Autodesk Fusion 360 part; units mm, degrees
sketch "Sketch1" plane through (0, 0, 0) normal (0, 0, 1) x (1, 0, 0)
  line L0 (-27.5, 0) -> (-12.5, 0)
  line L1 (-12.5, 0) -> (-12.5, 14.8)
  line L2 (-12.5, 14.8) -> (0, 14.8)
  line L3 (0, 31) -> (0, -29)
  line L4 (27.5, 0) -> (12.5, 0)
  line L5 (12.5, 0) -> (12.5, 14.8)
  line L6 (12.5, 14.8) -> (0, 14.8)
  line L7 (-27.5, 4) -> (-16.5, 4)
  line L8 (-16.5, 4) -> (-16.5, 18.8)
  line L9 (-16.5, 18.8) -> (0, 18.8)
  line L10 (16.5, 18.8) -> (0, 18.8)
  line L11 (16.5, 4) -> (16.5, 18.8)
  line L12 (27.5, 4) -> (16.5, 4)
  line L13 (27.5, 4) -> (27.5, 0)
  line L14 (-27.5, 4) -> (-27.5, 0)
  dimension "d2" = 4
  dimension "d3" = 15
  dimension "d4" = 25
  dimension "d5" = 14.8
extrude "Extrude1" add sketch "Sketch1" along normal blind 8
hole "Hole1" at (22.4998, 0, 3.8936) direction (0, 1, 0) diameter 4 depth 5 tip angle 118
hole "Hole2" at (-22.5548, 0, 4.1194) direction (0, 1, 0) diameter 4 depth 5 tip angle 118
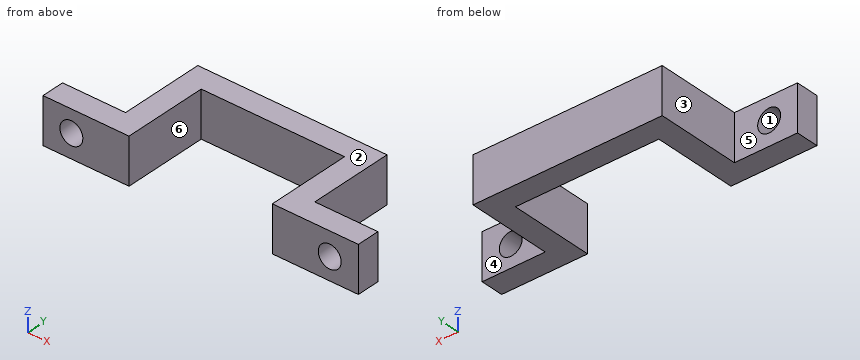
Verification items for the finished model (mm, model axes). Face numbers are marked on the shaded views. A direction names the side the tool comes from. Round coordinates to 2 decimals unless told otherwise and drop trailing zeros. Order: outer loops, then holes, each group sorted by start corner. A loop starts at its lowest first (then second) coordinate and runs counter-clockwise, first axis right, second up. Notation, with made-up numbers: (17.25, 70) - (24.25, 70) arc R8 cw to (24.25, 74) - close; hole circle Ø10 at (21.5, 25.5). An arc over 180 degrees is marked (long way). Use CSV: the item, a comma, the result in double quotes. Start each with the question number.
1) Go/stop test with flat-tipped pins: P1, Ø2.5, axis at x = 1, z = 5.5, coming from the -Y side; P2, Ø1.5, axis at x = 20, z = 6, coming from the +Y side; P3, Ø4, axis at y = 7.5, z = 4.5, coming from the +X side. Record where each tip stops, or that it passes through.
2) Access from +Z, -Z, +X, -X, +Y, -Y to the whole of each face (thin tool, end or side, straight path). Record for the marked faces 4, 5 and 6.
3) Thickness scan on L1, parallel to X at y = 6.5, z = 7.5; L2, parallel to X at y = 2.5, z = 7; L3, parallel to X at y = 1, z = 5.25. Record the ranges inside material, lowest first.
4) Section check A-A, the plane y = 7. Record the cut outline in (x, z), plus the area to 3 significant figures.
5) Section check D-D, the plane z = 3.5. Record the cut outline in (x, y).
6) Section check C-C, the plane x = 23.5. Record the cut outline in (y, z).
7) Section check B-B, the plane y = 1.5. Record the cut outline in (x, z).
8) Mould release check, pull along X, two halves, no side actions. Record for the marked faces 1, 2 and 3: +X half, -X half, draft (parallel to the pull), parting line (faces both ways), or undercut.
Answers:
1,P1,"stops at y = 14.8"
1,P2,"stops at y = 4"
1,P3,"stops at x = 16.5"
2,face 4,"+Z, -Z, +X, +Y"
2,face 5,"+Z, -Z, -X, +Y"
2,face 6,"+Z, -Z, -Y"
3,L1,"x = -16.5 to -12.5, 12.5 to 16.5"
3,L2,"x = -27.5 to -12.5, 12.5 to 27.5"
3,L3,"x = -27.5 to -24.2, -20.91 to -12.5, 12.5 to 21.03, 23.97 to 27.5"
4,outline,"(-16.5, 0) - (-12.5, 0) - (-12.5, 8) - (-16.5, 8) - close; (12.5, 0) - (16.5, 0) - (16.5, 8) - (12.5, 8) - close"
4,area,"64.0 mm²"
5,outline,"(-27.5, 0) - (-24.46, 0) - (-24.46, 4) - (-27.5, 4) - close; (-20.65, 0) - (-12.5, 0) - (-12.5, 14.8) - (12.5, 14.8) - (12.5, 0) - (20.54, 0) - (20.54, 4) - (16.5, 4) - (16.5, 18.8) - (-16.5, 18.8) - (-16.5, 4) - (-20.65, 4) - close; (24.46, 0) - (27.5, 0) - (27.5, 4) - (24.46, 4) - close"
6,outline,"(0, 0) - (4, 0) - (4, 2.16) - (0, 2.16) - close; (0, 5.63) - (4, 5.63) - (4, 8) - (0, 8) - close"
7,outline,"(-27.5, 0) - (-12.5, 0) - (-12.5, 8) - (-27.5, 8) - close; (12.5, 0) - (27.5, 0) - (27.5, 8) - (12.5, 8) - close; hole circle Ø4 at (-22.55, 4.12); hole circle Ø4 at (22.5, 3.89)"
8,face 1,"undercut"
8,face 2,"draft"
8,face 3,"-X half"
